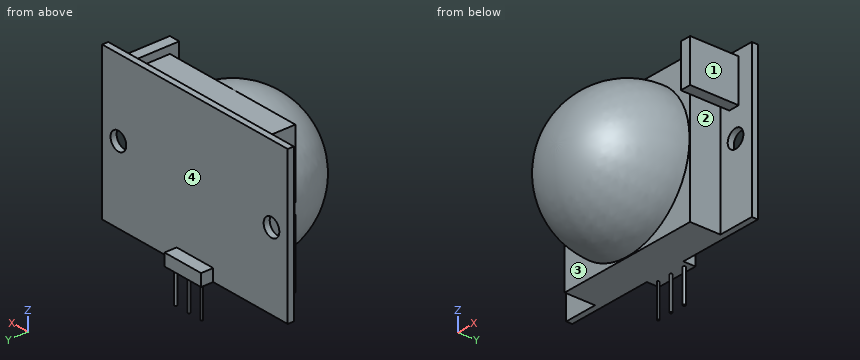
from build123d import *

# Parameters (mm, degrees)
F0_W      = 35.5
F0_H      = 25
F1_DEPTH  = 1
F2_W      = 24
F2_H      = 24
F3_DEPTH  = 5
F7_W      = 1.8
F7_H      = 7
F8_DEPTH  = 8
F9_R      = 1.5
F10_DEPTH = 25
F11_W     = 7
F11_H     = 2
F12_DEPTH = 2
F13_R     = 0.2
F13_R_2   = 0.180913
F13_R_3   = 0.154128
F14_DEPTH = 5.5


with BuildPart() as f1:
    # F0 (on Front) → F1 (new body)
    with BuildSketch(Plane.XZ):
        Rectangle(F0_W, F0_H)
    extrude(amount=-F1_DEPTH)

    # F2 (on face) → F3 (join)
    with BuildSketch(Plane.XZ):
        with Locations((-0.25, -0.5)):
            Rectangle(F2_W, F2_H)
    extrude(amount=F3_DEPTH)

    # F5 (on offset) → F6 (revolve)
    with BuildSketch(Plane.XY.offset(-0.5)):
        with BuildLine():
            ThreePointArc((-0.25, -16.9), (8.164571, -13.414571), (11.65, -5))
            Line((11.65, -5), (-0.25, -5))
            Line((-0.25, -5), (-0.25, -16.9))
        make_face()
    revolve(axis=Axis((-0.25, -10.95, -0.5), (0, -1, 0)))

    # F7 (on face) → F8 (join)
    with BuildSketch(Plane.XZ):
        with Locations((14.35, 8)):
            Rectangle(F7_W, F7_H)
    extrude(amount=F8_DEPTH)

    # F9 (on face) → F10 (cut)
    with BuildSketch(Plane.XZ):
        with Locations((-14.65, 0)):
            Circle(F9_R)
        with Locations((14.65, 0)):
            Circle(F9_R)
    extrude(amount=-F10_DEPTH, mode=Mode.SUBTRACT)

    # F11 (on face) → F12 (join)
    with BuildSketch(Plane(origin=(0, 1, 0), x_dir=(-1, 0, 0), z_dir=(0, 1, 0))):
        with Locations((0, -11.5)):
            Rectangle(F11_W, F11_H)
    extrude(amount=F12_DEPTH)

    # F13 (on face) → F14 (join)
    with BuildSketch(Plane(origin=(0, 0, -12.5), x_dir=(1, 0, 0), z_dir=(0, 0, -1))):
        with Locations((2.5, -2)):
            Circle(F13_R)
        with Locations((0, -2)):
            Circle(F13_R_2)
        with Locations((-2.5, -2)):
            Circle(F13_R_3)
    extrude(amount=F14_DEPTH)


solid = f1.part
Geometry: final body of the model. Coordinates: model frame, mm. Face numbers are marked on the shaded views. Give positions to 0.01 mm unless a question says otherwise; leave off trailing zeros. Order: outer loops, then holes, each group sorted by start corner. A loop starts at its lowest first (then second) coordinate and runs counter-clockwise, first axis right, second up. Notation, with made-up numbers: (89.5, 77.25) -> (97.5, 77.25) arc R33 ccw to (97.5, 105.25) -> close; hole circle Ø5 at (29.25, 72). An arc over 180 degrees is marked (long way). Write each question's results on one line, items separated by ' | '.
1) Cut plane C-C (z = 0.5). Give the number of separate pieces and of enclosed holes in the cut face, and give its area (3 significant figures).
Geometry says:
separate pieces: 3 | enclosed holes: 0 | area: 371 mm²
2) Cut plane A-A (x = -14.65). Output: boundary loops of the cut face in (y, z), and give its area (3 significant figures).
Geometry says:
outline: (0, -12.5) -> (1, -12.5) -> (1, -1.5) -> (0, -1.5) -> close; (0, 1.5) -> (1, 1.5) -> (1, 12.5) -> (0, 12.5) -> close | area: 22.0 mm²
3) First-contact query: pin 1 Ø1 at (x, z) = (0, -9.5) entering from +Y; pin 2 Ø0.9 at (x, y) = (14.5, -2) entering from -Z; pin 3 Ø4 at (x, y) = (-6.5, -13.5) entering from +Z. Flat tips, straight axial feed; report the tip coordinate or a pass-through.
Geometry says:
pin 1: stops at y = 1 | pin 2: stops at z = 4.5 | pin 3: stops at z = 7.78
4) Cut plane B-B (z = -13). Output: boundary loops of the cut face in (x, y).
Geometry says:
outline: circle Ø0.31 at (-2.5, 2); circle Ø0.36 at (0, 2); circle Ø0.4 at (2.5, 2)
5) Line query: line 1 along Z through (x, y) = (14.65, 0.6); line 2 along X through (y, z) = (-4.75, 10.5); line 3 along Y through (x, z) = (14, -3.5). Output: solid intervals per line, ascending.
Geometry says:
line 1: z = -12.5 to -1.5, 1.5 to 12.5 | line 2: x = -12.25 to 11.75, 13.45 to 15.25 | line 3: y = 0 to 1
6) Draft query along X for the marked faces 1, 2, 3 and 4. Return one class per face: released by +X, released by -X, zero draft, split by the parting line, or undercut.
Geometry says:
face 1: released by +X | face 2: undercut | face 3: undercut | face 4: zero draft
